For this review, use the dimensioned drawing (mm, ordinates from the lowest corner) and the shaded views. Coordinates: 2 decimals unless noted, no trailing zeros. Loops run counter-clockwise (first coordinate to the right, second up) from the corner with the lowest first, then second, coordinate; pieces in that order, holes last. Notation, with made-up numbers: (34.5, -12) -> (59.5, -12) arc R32 cw to (59.5, 23) -> close; hole circle Ø6 at (71.25, -17). An arc over 180 degrees is marked (long way). Use one line per item in the form item = value. Start each with the question number.
1. Wall thickness on line 1 (Y direction, x = 4.5, z = 3.2); line 2 (Y direction, x = 5, z = 0.25); line 3 (X direction, y = 4.25, z = 0.25): over which ranges is each line inside the solid? List them lowest first. Write a range as from..to.
2. Consider section A-A (x = 4.5). State the section outline as (y, z) points.
3. The part is to be moulded in two halves that separate along Y. For the marked faces 1, 2 and 3, say which applies: released by +Y, released by -Y, zero draft, split by the parting line, or undercut.
4. Consider section B-B (z = 3.3). State the section outline as (x, y) points.
5. For pin 1 (1 mm diameter, centred on x = 2.5, z = 4, fed in from +Y); pin 2 (5 mm diameter, centred on x = 4.5, y = 7.5, fed in from -Z); pin 3 (2 mm diameter, centred on y = 2.5, z = 3.5, fed in from -X); pin 4 (1.8 mm diameter, centred on x = 4.5, y = 4.5, fed in from +Z), all flat-tipped, find the tip position at first contact; note any pin that passes through.
6. Consider section C-C (z = 0.8). State the section outline as (x, y) points.
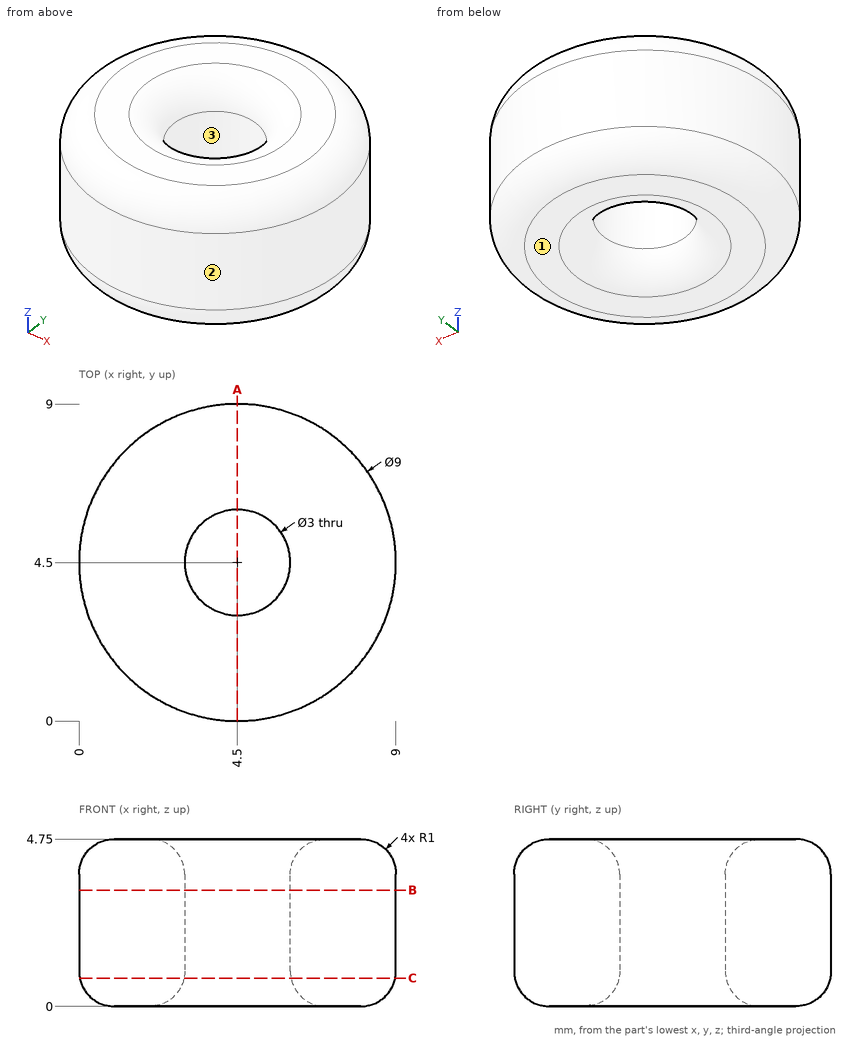
Geometry check:
q1.line_1 = 0..3, 6..9
q1.line_2 = 0.37..2.73, 6.27..8.63
q1.line_3 = 0.35..2.68, 6.32..8.65
q2.outline = (0, 1) arc R1 ccw to (1, 0) -> (2, 0) arc R1 ccw to (3, 1) -> (3, 3.75) arc R1 ccw to (2, 4.75) -> (1, 4.75) arc R1 ccw to (0, 3.75) -> close; (6, 1) arc R1 ccw to (7, 0) -> (8, 0) arc R1 ccw to (9, 1) -> (9, 3.75) arc R1 ccw to (8, 4.75) -> (7, 4.75) arc R1 ccw to (6, 3.75) -> close
q3.face_1 = zero draft
q3.face_2 = split by the parting line
q3.face_3 = undercut
q4.outline = circle Ø9 at (4.5, 4.5); hole circle Ø3 at (4.5, 4.5)
q5.pin_1 = 8.73
q5.pin_2 = 0
q5.pin_3 = 0.11
q5.pin_4 = through
q6.outline = circle Ø8.96 at (4.5, 4.5); hole circle Ø3.04 at (4.5, 4.5)
